from build123d import *

# Parameters (mm, degrees)
BOSS_EXTRUDE1_DEPTH = 3.175
SKETCH2_R           = 9.946432709
SKETCH2_R_2         = 8.628774031
SKETCH2_R_3         = 7.9375
SKETCH2_R_4         = 7.14375
CUT_EXTRUDE1_DEPTH  = 4.175


with BuildPart() as part:
    # Sketch1 → Boss-Extrude1 (new body)
    with BuildSketch(Plane.XY):
        Polygon((0, 0), (50.8, 0), (60, -37.754085603), (60, -69.85), (-41.787887726, -69.85), (-138.966701689, -78.087543548), (-169.514196693, -118.67683461), (-199.95616499, -95.766213357), (-169.408669986, -55.176922294), (-42.8625, -44.45), (0, -44.45), align=None)
    extrude(amount=BOSS_EXTRUDE1_DEPTH)

    # Sketch2 → Cut-Extrude1 (cut, through all)
    with BuildSketch(Plane.XY.offset(3.175)):
        with Locations((-171.31481468, -84.35191449)):
            Circle(SKETCH2_R)
        with Locations((-152.715034722, -66.714192116)):
            Circle(SKETCH2_R_2)
        with Locations((-125.957448531, -64.239244165)):
            Circle(SKETCH2_R_3)
        with Locations((-103.811868784, -62.362032763)):
            Circle(SKETCH2_R_3)
        with Locations((-81.666289037, -60.484821362)):
            Circle(SKETCH2_R_3)
        with Locations((-59.52070929, -58.60760996)):
            Circle(SKETCH2_R_3)
        with Locations((-37.375129542, -56.730398559)):
            Circle(SKETCH2_R_3)
        with Locations((-11.455180712, -57.15)):
            Circle(SKETCH2_R_4)
        with Locations((10.769819288, -57.15)):
            Circle(SKETCH2_R_4)
        with Locations((32.994819288, -57.15)):
            Circle(SKETCH2_R_4)
        with Locations((10.769819288, -34.925)):
            Circle(SKETCH2_R_4)
        with Locations((32.994819288, -34.925)):
            Circle(SKETCH2_R_4)
        with Locations((10.769819288, -12.7)):
            Circle(SKETCH2_R_4)
        with Locations((32.994819288, -12.7)):
            Circle(SKETCH2_R_4)
        with Locations((-11.455180712, -34.925)):
            Circle(SKETCH2_R_4)
        with Locations((-11.455180712, -12.7)):
            Circle(SKETCH2_R_4)
        with Locations((50.457319288, -34.925)):
            Circle(SKETCH2_R_4)
    extrude(amount=-CUT_EXTRUDE1_DEPTH, mode=Mode.SUBTRACT)


solid = part.part
Build history of the part. All positions in model axes, mm. Coordinates: 2 decimals unless noted, no trailing zeros. Order: outer loops, then holes, each group sorted by start corner. A loop starts at its lowest first (then second) coordinate and runs counter-clockwise, first axis right, second up. Notation, with made-up numbers: (-25.75, -16) - (27.25, -16) arc R29 ccw to (27.25, 7) - close; hole circle Ø5 at (78, 4.5). An arc over 180 degrees is marked (long way). Write item = value, one per line. Start each with the question number.
1) Flat gauge pins, fed straight in: pin 1 Ø9.5 at (x, y) = (-81.67, -60.48) entering from +Z (3 decimals); pin 2 Ø23 at (x, y) = (-171.31, -84.35) entering from +Z (3 decimals); pin 3 Ø1 at (y, z) = (-33.5, 2.5) entering from +X; pin 4 Ø1 at (x, z) = (-16, 1) entering from -Y. Where does each tip first touch, or does it go through?
2) Saw through at C-C on y = -12.7. Write the cut outline in (x, z) (3 decimals), then the cut area to 3 significant figures.
3) Two-plate mould, pull along X, no slides. Class faces 1 (the face through (-96.24, -59.98, 1.61)), 2 (the face through (-154.03, -98.1, 1.57)), 3 (the face through (-184.9, -75.76, 1.57)): pulls with the +X half, pulls with the -X half, needs draft (parallel to the pull), parting line crosses it, or undercut.
4) Saw through at D-D on x = -123. Write the cut outline in (y, z) (3 decimals), then the cut area to 3 significant figures.
5) Saw through at B-B on z = 1.1. Count the separate pieces of the cut face and the enclosed holes in it, then the cut area to 3 significant figures.
6) Wall check: line 1 along X through (y, z) = (-9, 2.65); line 2 along X through (y, z) = (-36, 0.7); line 3 along X through (y, z) = (-65.5, 0.65). Give the ranges that are in metal, low to high. Write a range as from..to.
7) Saw through at A-A on x = 31.5. Write the cut outline in (y, z) (3 decimals).
From the geometry:
q1.pin_1 = through
q1.pin_2 = 3.175
q1.pin_3 = 59.09
q1.pin_4 = -69.85
q2.outline = (0, 0) - (3.626, 0) - (3.626, 3.175) - (0, 3.175) - close; (17.914, 0) - (25.851, 0) - (25.851, 3.175) - (17.914, 3.175) - close; (40.139, 0) - (53.895, 0) - (53.895, 3.175) - (40.139, 3.175) - close
q2.area = 80.4 mm^2
q3.face_1 = undercut
q3.face_2 = pulls with the +X half
q3.face_3 = pulls with the -X half
q4.outline = (-76.734, 0) - (-71.605, 0) - (-71.605, 3.175) - (-76.734, 3.175) - close; (-56.873, 0) - (-51.243, 0) - (-51.243, 3.175) - (-56.873, 3.175) - close
q4.area = 34.2 mm^2
q5.separate_pieces = 1
q5.enclosed_holes = 15
q5.area = 7,060 mm^2
q6.line_1 = 0..4.66, 16.88..26.88, 39.11..52.99
q6.line_2 = 0..3.71, 17.83..25.93, 40.06..43.39, 57.52..59.57
q6.line_3 = -177.18..-161.26, -144.17..-133.79, -118.12..-111.1, -96.52..-87.82, -75.51..-63.46, -55.58..60
q7.outline = (-69.85, 0) - (-64.136, 0) - (-64.136, 3.175) - (-69.85, 3.175) - close; (-50.164, 0) - (-41.911, 0) - (-41.911, 3.175) - (-50.164, 3.175) - close; (-27.939, 0) - (-19.686, 0) - (-19.686, 3.175) - (-27.939, 3.175) - close; (-5.714, 0) - (0, 0) - (0, 3.175) - (-5.714, 3.175) - close
